Source: three-view drawing plus pictorial views. Frame: mm from the lowest corner of the part. Round coordinates to 2 decimals unless told otherwise and drop trailing zeros. Loops run counter-clockwise (first coordinate to the right, second up) from the corner with the lowest first, then second, coordinate; pieces in that order, holes last. Notation, with made-up numbers: (-22, -10.75) -> (1, -10.75) arc R30 cw to (1, 12.25) -> close; hole circle Ø4 at (45.5, 75). An arc over 180 degrees is marked (long way). Put each result on its own line as item: value. Start each with the question number.
1. Cut plane C-C (z = 8.25). Return the cut outline in (x, y), then the cut area to 3 significant figures.
2. Cut plane D-D (z = 1). Return the cut outline in (x, y) (3 decimals), then the cut area to 3 significant figures.
3. Contact query for flat-ended pins moving along their axis: pin 1 (1.6 mm diameter, centred on x = 17.5, z = 1.5, fed in from -Y) (3 decimals); pin 2 (3.5 mm diameter, centred on x = 24.5, z = 1, fed in from +Y) (3 decimals); pin 3 (3.5 mm diameter, centred on y = 16, z = 1, fed in from -X) (3 decimals). Output: stop coordinate, or through.
4. Cut plane A-A (y = 6). Return the cut outline in (x, z) (3 decimals).
5. Material intervals for L1, parallel to Y at x = 37.5, z = 2.25 (3 decimals); L2, parallel to Y at x = 5, z = 9.25, sorted ascending.
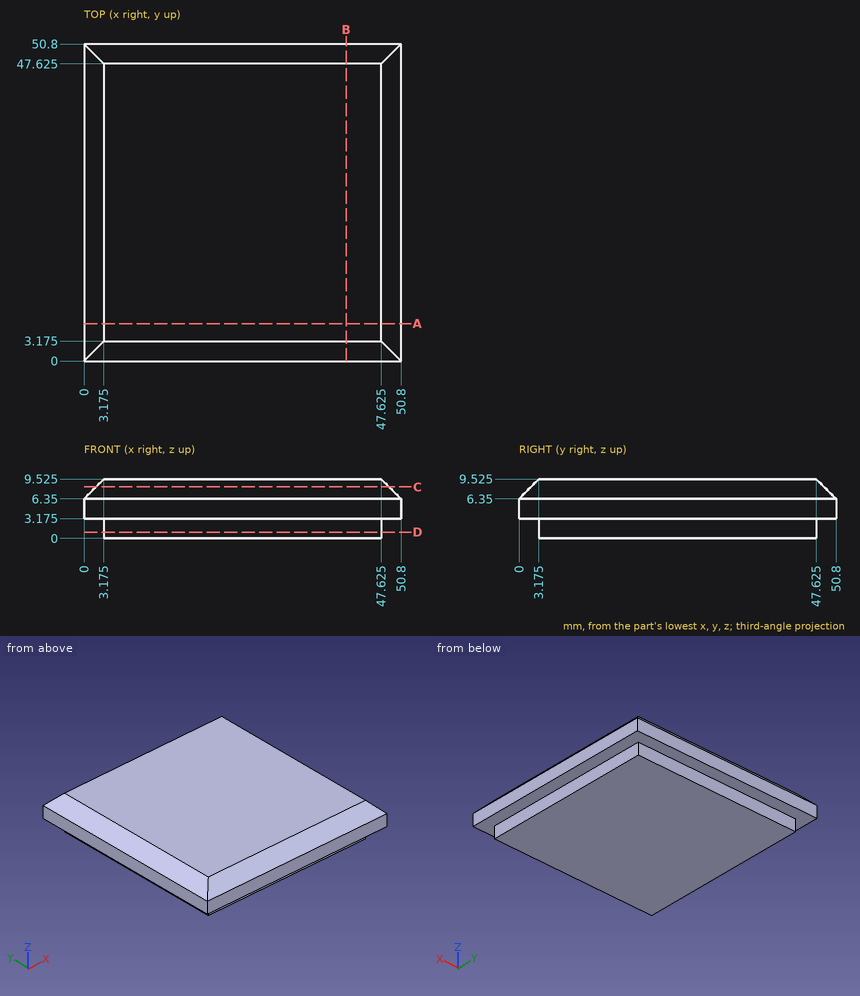
Solution:
1. outline: (1.9, 1.9) -> (48.9, 1.9) -> (48.9, 48.9) -> (1.9, 48.9) -> close
1. area: 2,210 mm^2
2. outline: (3.175, 3.175) -> (47.625, 3.175) -> (47.625, 47.625) -> (3.175, 47.625) -> close
2. area: 1,980 mm^2
3. pin 1: stops at y = 3.175
3. pin 2: stops at y = 47.625
3. pin 3: stops at x = 3.175
4. outline: (0, 3.175) -> (3.175, 3.175) -> (3.175, 0) -> (47.625, 0) -> (47.625, 3.175) -> (50.8, 3.175) -> (50.8, 6.35) -> (47.625, 9.525) -> (3.175, 9.525) -> (0, 6.35) -> close
5. L1: y = 3.175 to 47.625
5. L2: y = 2.9 to 47.9
